Geometry: final body of the model. Coordinates: model frame, mm. Face numbers are marked on the shaded views. A direction names the side the tool comes from. Coordinates: 2 decimals unless noted, no trailing zeros. Write each loop counter-clockwise with the first axis right and the second up, starting at its lowest first coordinate (ties: lowest second). Pieces come first, ordered by that corner, then holes. Notation, with made-up numbers: (54.5, -5) - (69.5, -5) arc R25 cw to (69.5, 23) - close; hole circle Ø3 at (65, 38.25). An arc over 180 degrees is marked (long way). Answer as a JSON object with one key per item and string values. Group by question number.
Item 1: Section A-A on z = 0. Return loops of the section in (x, y), and give its area (3 significant figures).
Item 2: First-contact query: pin 1 Ø4 at (x, y) = (-6, -38) entering from +Z (3 decimals); pin 2 Ø4 at (x, y) = (10, -27.5) entering from -Z; pin 3 Ø8 at (x, z) = (9.5, -17.5) entering from +Y. Flat tips, straight axial feed; report the tip coordinate or a pass-through.
Item 3: Set-up query: the marked faces 3 and 4. Return all of +Z, -Z, +X, -X, +Y, -Y with unobstructed straight access to the full face (end or side cutting, diameter ignored); none if empty.
Item 4: Mould query, pull axis Z, two halves, no side actions, for the marked faces 1 and 2. Classes: pulls with the +Z half, pulls with the -Z half, needs draft (parallel to the pull), parting line crosses it, or undercut.
Item 5: Section B-B on x = 0. Return loops of the section in (y, z).
Item 6: Section C-C on y = -2. Return loops of the section in (x, z).
Item 7: Line query: line 1 along Z through (x, y) = (16, -0.5); line 2 along Y through (x, z) = (-18.5, 18); line 3 along Y through (x, z) = (-14.5, 15). Output: solid intervals per line, ascending. Write a range as from..to.
Item 8: Section D-D on y = -11.5. Return loops of the section in (x, z), and give its area (3 significant figures).
```python
from build123d import *

# Parameters (mm, degrees)
F0_R     = 31.5
F0_R_2   = 2
F0_R_3   = 4
F1_DEPTH = 66
F2_DEPTH = 27
F3_DEPTH = 10
F4_SIZE2 = 3.5
F4_SIZE  = 10
F5_SIZE2 = 10
F5_SIZE  = 3.5
F6_R     = 7.75
F6_R_2   = 4
F7_DEPTH = 2


with BuildPart() as f1:
    # F0 (on Front) → F1 (new body)
    with BuildSketch(Plane.XZ):
        Circle(F0_R)
        with Locations((-15.5563491861, -15.5563491861)):
            Circle(F0_R_2, mode=Mode.SUBTRACT)
        with Locations((15.5563491861, -15.5563491861)):
            Circle(F0_R_2, mode=Mode.SUBTRACT)
        with Locations((-15.5563491861, 15.5563491861)):
            Circle(F0_R_2, mode=Mode.SUBTRACT)
        Circle(F0_R_3, mode=Mode.SUBTRACT)
        with Locations((15.5563491861, 15.5563491861)):
            Circle(F0_R_2, mode=Mode.SUBTRACT)
        Circle(F0_R_3)
        with Locations((15.5563491861, 15.5563491861)):
            Circle(F0_R_2)
        with Locations((-15.5563491861, 15.5563491861)):
            Circle(F0_R_2)
        with Locations((-15.5563491861, -15.5563491861)):
            Circle(F0_R_2)
        with Locations((15.5563491861, -15.5563491861)):
            Circle(F0_R_2)
    extrude(amount=F1_DEPTH)

    # F0 (on Front) → F2 (join)
    with BuildSketch(Plane.XZ):
        Circle(F0_R_3)
    extrude(amount=-F2_DEPTH)

    # F0 (on Front) → F3 (cut)
    with BuildSketch(Plane.XZ):
        with Locations((15.5563491861, 15.5563491861)):
            Circle(F0_R_2)
        with Locations((-15.5563491861, 15.5563491861)):
            Circle(F0_R_2)
        with Locations((15.5563491861, -15.5563491861)):
            Circle(F0_R_2)
        with Locations((-15.5563491861, -15.5563491861)):
            Circle(F0_R_2)
    extrude(amount=F3_DEPTH, mode=Mode.SUBTRACT)

    # F4
    f4_edges = [f1.edges().sort_by_distance(p)[0] for p in [
        (-31.5, 0, 0),
    ]]
    f4_side = f1.faces().sort_by_distance((-31.5, -33, 0))[0]
    chamfer(f4_edges, length=F4_SIZE, length2=F4_SIZE2, reference=f4_side)

    # F5
    f5_edges = [f1.edges().sort_by_distance(p)[0] for p in [
        (-31.5, -66, 0),
    ]]
    f5_side = f1.faces().sort_by_distance((0, -66, 0))[0]
    chamfer(f5_edges, length=F5_SIZE, length2=F5_SIZE2, reference=f5_side)

    # F6 (on face) → F7 (join)
    with BuildSketch(Plane(origin=(0, 0, 0), x_dir=(-1, 0, 0), z_dir=(0, 1, 0))):
        Circle(F6_R)
        Circle(F6_R_2, mode=Mode.SUBTRACT)
    extrude(amount=F7_DEPTH)


solid = f1.part
```
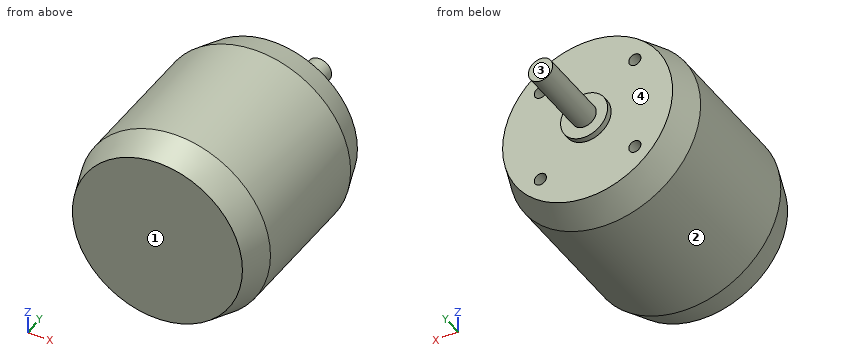
Checks:
{
 "1": {"outline": "(-31.5, -56) - (-28, -66) - (28, -66) - (31.5, -56) - (31.5, -10) - (28, 0) - (7.75, 0) - (7.75, 2) - (4, 2) - (4, 27) - (-4, 27) - (-4, 2) - (-7.75, 2) - (-7.75, 0) - (-28, 0) - (-31.5, -10) - close", "area": "4,320 mm^2"},
 "2": {"pin 1": "z = 31.245", "pin 2": "z = -30.47", "pin 3": "y = 0"},
 "3": {"face 3": "+Z, -Z, +X, -X, +Y", "face 4": "+Y"},
 "4": {"face 1": "needs draft", "face 2": "parting line crosses it"},
 "5": {"outline": "(-66, -28) - (-56, -31.5) - (-10, -31.5) - (0, -28) - (0, -7.75) - (2, -7.75) - (2, -4) - (27, -4) - (27, 4) - (2, 4) - (2, 7.75) - (0, 7.75) - (0, 28) - (-10, 31.5) - (-56, 31.5) - (-66, 28) - close"},
 "6": {"outline": "circle Ø57.4 at (0, 0); hole circle Ø4 at (-15.56, -15.56); hole circle Ø4 at (-15.56, 15.56); hole circle Ø4 at (15.56, -15.56); hole circle Ø4 at (15.56, 15.56)"},
 "7": {"line 1": "-23.19..-17.51, -13.61..13.61, 17.51..23.19", "line 2": "-66..0", "line 3": "-66..-10"},
 "8": {"outline": "circle Ø63 at (0, 0)", "area": "3,120 mm^2"}
}
